Design review of the part built by this model. Coordinates are the model's own, in mm. Give positions to 0.01 mm unless a question says otherwise; leave off trailing zeros. Order: outer loops, then holes, each group sorted by start corner. A loop starts at its lowest first (then second) coordinate and runs counter-clockwise, first axis right, second up. Notation, with made-up numbers: (75.5, 13.25) -> (89.5, 13.25) arc R29 ccw to (89.5, 36.25) -> close; hole circle Ø9 at (70.5, 74). An arc over 180 degrees is marked (long way). One line per item, written item: value. Start each with the question number.
1) Consider section B-B (z = 0). State the section outline as (x, y) points, plus the area to 3 significant figures.
2) Consider section A-A (z = 25.4). State the section outline as (x, y) points.
3) Wall thickness on line 1 along Y through (x, z) = (2.5, 0); line 2 along Y through (x, z) = (4, 25): over which ranges is each line inside the solid? List them lowest first. Write a range as from..to.
4) The part is to be moulded in two halves that separate along Y. For faces 1 (the face through (-0.07, -134.81, 24.05)), 2 (the face through (0, -161, 38.1)), 3 (the face through (0, -91.694, 13)), say which applies: released by +Y, released by -Y, zero draft, split by the parting line, or undercut.
from build123d import *

# Parameters (mm, degrees)
SKETCH1_W             = 50.8
SKETCH1_H             = 136.906
SKETCH1_R             = 3.925
BOSS_EXTRUDE1_DEPTH   = 4.7625
F_6_32_TAPPED_HOLE1_D = 2.7051


with BuildPart() as part:
    # Sketch1 → Boss-Extrude1 (new, symmetric)
    with BuildSketch(Plane(origin=(0, 0, 0), x_dir=(0, 0, -1), z_dir=(1, 0, 0))):
        with Locations((-12.7, -160.147)):
            Rectangle(SKETCH1_W, SKETCH1_H)
        with Locations((0, -115.824)):
            Circle(SKETCH1_R, mode=Mode.SUBTRACT)
    extrude(amount=BOSS_EXTRUDE1_DEPTH, both=True)

    # #6-32 Tapped Hole1 (through all)
    with Locations(Plane(origin=(4.7625, 0, 0), x_dir=(0, 0, -1), z_dir=(1, 0, 0))):
        with Locations((-25.4, -96.774), (0, -96.774), (0, -134.874), (-25.4, -134.874)):
            Hole(F_6_32_TAPPED_HOLE1_D / 2)


solid = part.part
Checked values:
1. outline: (-4.76, -228.6) -> (4.76, -228.6) -> (4.76, -136.23) -> (-4.76, -136.23) -> close; (-4.76, -133.52) -> (4.76, -133.52) -> (4.76, -119.75) -> (-4.76, -119.75) -> close; (-4.76, -111.9) -> (4.76, -111.9) -> (4.76, -98.13) -> (-4.76, -98.13) -> close; (-4.76, -95.42) -> (4.76, -95.42) -> (4.76, -91.69) -> (-4.76, -91.69) -> close
1. area: 1,180 mm^2
2. outline: (-4.76, -228.6) -> (4.76, -228.6) -> (4.76, -136.23) -> (-4.76, -136.23) -> close; (-4.76, -133.52) -> (4.76, -133.52) -> (4.76, -98.13) -> (-4.76, -98.13) -> close; (-4.76, -95.42) -> (4.76, -95.42) -> (4.76, -91.69) -> (-4.76, -91.69) -> close
3. line 1: y = -228.6..-136.23, -133.52..-119.75, -111.9..-98.13, -95.42..-91.69
3. line 2: y = -228.6..-136.17, -133.58..-98.07, -95.48..-91.69
4. face 1: undercut
4. face 2: zero draft
4. face 3: released by +Y
